Geometry: final body of the model. Coordinates: model frame, mm. A direction names the side the tool comes from. Give positions to 0.01 mm unless a question says otherwise; leave off trailing zeros. Order: outer loops, then holes, each group sorted by start corner. A loop starts at its lowest first (then second) coordinate and runs counter-clockwise, first axis right, second up. Notation, with made-up numbers: (-9, 37) -> (24, 37) arc R7 ccw to (24, 45) -> close; hole circle Ø10 at (41, 27.25). An arc over 180 degrees is marked (long way). Write item = value, one per line.
Autodesk Inventor part; units mm, degrees
ref_plane "YZ Plane" through (0, 0, 0) normal (1, 0, 0) x (0, 1, 0)
ref_plane "XZ Plane" through (0, 0, 0) normal (0, 1, 0) x (-1, 0, 0)
ref_plane "XY Plane" through (0, 0, 0) normal (0, 0, 1) x (1, 0, 0)
sketch "Boceto1" plane through (0, 0, 0) normal (0, 0, 1) x (1, 0, 0)
  line L0 (-8, 35) -> (8, 35)
  line L1 (8, 35) -> (8, -35)
  line L2 (8, -35) -> (-8, -35)
  line L3 (-8, -35) -> (-8, 35)
  line L4 (-8, 35) -> (8, -35) construction
  line L5 (8, 35) -> (-8, -35) construction
  point P0 (0, 0)
  dimension "d0" = 16
  dimension "d1" = 70
extrude "Extrusión1" add sketch "Boceto1" along normal blind 2
sketch "Boceto2" plane through (0, 0, 2) normal (0, 0, 1) x (1, 0, 0)
  line L0 (38, -62.5) -> (8, -62.5)
  line L1 (8, -62.5) -> (8, 62.5)
  line L2 (8, 62.5) -> (38, 62.5)
  line L3 (38, 62.5) -> (38, -62.5)
  line L4 (38, -62.5) -> (8, 62.5) construction
  line L5 (8, -62.5) -> (38, 62.5) construction
  point P0 (0, 0)
  point P1 (23, 0)
  dimension "d4" = 30
  dimension "d5" = 125
extrude "Extrusión2" add sketch "Boceto2" against normal blind 30
sketch "Boceto3" plane through (0, 0, 2) normal (0, 0, 1) x (1, 0, 0)
  line L0 (38, 62.5) -> (38, -62.5)
  line L1 (13.5714, -44.7856) -> (13.5714, 45.755)
  line L2 (38, 45.755) -> (38, -44.7856)
  line L3 (13.5714, -44.7856) -> (38, -52.7345)
  line L4 (38, -52.7345) -> (38, -44.7856)
  line L5 (13.5714, 45.755) -> (38, 53.8978)
  line L6 (38, 45.755) -> (38, 53.8978)
  line L7 (8, -62.5) -> (8, -35)
  line L8 (38, -62.5) -> (8, -62.5)
  line L9 (8, -62.5) -> (38, -62.5)
  line L10 (38, -62.5) -> (8, -52.7345)
  line L11 (8, -52.7345) -> (8, -62.5)
  line L12 (8, -62.5) -> (8, 62.5)
  line L13 (8, 62.5) -> (38, 62.5)
  line L14 (38, 62.5) -> (8, 52.5)
  line L15 (8, 62.5) -> (38, 62.5)
  line L16 (8, 52.5) -> (8, 62.5)
  point P0 (0, 0)
extrude "Extrusión3" cut sketch "Boceto3" against normal through all contours L14 L12 L13 | L0 L3 L1 L5 | L10 L8 L7
sketch "Boceto4" plane through (0, 0, 0) normal (0, 0, -1) x (-1, 0, 0)
  point P0 (0, 0)
  point P1 (0, 0)
  point P2 (0, 15)
  point P3 (0, 30)
  point P4 (0, -15)
  point P5 (0, -30)
hole "Agujero1" at (0, 0, 0) at (0, 15, 0) at (0, 30, 0) at (0, -15, 0) at (0, -30, 0) direction (0, 0, 1) diameter 3.175 end through all
properties part number "Pala"
1) Section query D-D (y = -49.5). Output: boundary loops of the cut face in (x, z).
Check sheet entries:
outline = (8, -28) -> (28.06, -28) -> (28.06, 2) -> (8, 2) -> close
2) Section query C-C (z = -12). Output: boundary loops of the cut face in (x, y) (1 decimal).
Check sheet entries:
outline = (8, -52.7) -> (38, -62.5) -> (38, -52.7) -> (13.6, -44.8) -> (13.6, 45.8) -> (38, 53.9) -> (38, 62.5) -> (8, 52.5) -> close
3) Reachability of faces 1 (the face through (25.615, 49.769, -12.79)), 2 (the face through (23.21, 57.57, -12.79)), 3 (the face through (-2, 0, 0)) from +Z, -Z, +X, -X, +Y, -Y: full face, straight path, thin tool, end or side. Return the list, or none.
Check sheet entries:
face_1 = +Z, -Z, +X
face_2 = +Z, -Z, -X, +Y
face_3 = -Z, -X, +Y, -Y
4) Section query A-A (y = 15). Output: boundary loops of the cut face in (x, z).
Check sheet entries:
outline = (-8, 0) -> (-1.59, 0) -> (-1.59, 2) -> (-8, 2) -> close; (1.59, 0) -> (8, 0) -> (8, -28) -> (13.57, -28) -> (13.57, 2) -> (1.59, 2) -> close
5) Line query: line 1 (Y direction, x = 0, z = 0.8); line 2 (X direction, y = 15, z = 0.7); line 3 (X direction, y = -5, z = -16.75). Output: solid intervals per line, ascending. Write a range as from..to.
Check sheet entries:
line_1 = -35..-31.59, -28.41..-16.59, -13.41..-1.59, 1.59..13.41, 16.59..28.41, 31.59..35
line_2 = -8..-1.59, 1.59..13.57
line_3 = 8..13.57
6) First-contact query: P1, Ø6, axis at x = 7, z = -2.5, coming from the +Y side; P2, Ø1.9, axis at x = 0, y = -15, coming from the +Z side; P3, Ø3, axis at x = 27.5, z = -7.5, coming from the -Y side; P4, Ø9, axis at y = -18.5, z = -8.5, coming from the -X side. Flat tips, straight axial feed; report the tip coordinate or a pass-through.
Check sheet entries:
P1 = 53.17
P2 = through
P3 = -59.57
P4 = 8
7) Section query B-B (x = 0). Output: boundary loops of the cut face in (y, z), plus the area to 3 significant figures.
Check sheet entries:
outline = (-35, 0) -> (-31.59, 0) -> (-31.59, 2) -> (-35, 2) -> close; (-28.41, 0) -> (-16.59, 0) -> (-16.59, 2) -> (-28.41, 2) -> close; (-13.41, 0) -> (-1.59, 0) -> (-1.59, 2) -> (-13.41, 2) -> close; (1.59, 0) -> (13.41, 0) -> (13.41, 2) -> (1.59, 2) -> close; (16.59, 0) -> (28.41, 0) -> (28.41, 2) -> (16.59, 2) -> close; (31.59, 0) -> (35, 0) -> (35, 2) -> (31.59, 2) -> close
area = 108 mm²
8) Mould query, pull axis X, two halves, no side actions, for faces 4 (the face through (-0.477, 31.514, 1.014)), 5 (the face through (10, 0, 2)), 6 (the face through (38, 58, -13)). Classes: +X half, -X half, draft (parallel to the pull), parting line (faces both ways), or undercut.
Check sheet entries:
face_4 = undercut
face_5 = draft
face_6 = +X half
